from build123d import *

# Parameters (mm, degrees)
F1_DEPTH = 289.46
F2_W     = 128
F2_H     = 8.4
F3_DEPTH = 7
F5_DEPTH = 289.46


with BuildPart() as f1:
    # F0 (on Front) → F1 (new body)
    with BuildSketch(Plane.XZ):
        Polygon((-47.436745, 38.990075), (-57.436745, 38.990075), (-57.436745, 36.490075), (-54.436745, 36.490075), (-54.436745, 33.090075), (-56.436745, 33.090075), (-56.436745, 30.590075), (-47.436745, 30.590075), align=None)
    extrude(amount=F1_DEPTH)

    # F2 (on Front) → F3 (join)
    with BuildSketch(Plane.XZ):
        with Locations((-111.436745, 34.790075)):
            Rectangle(F2_W, F2_H)
    extrude(amount=-F3_DEPTH)

    # F4 (on Front) → F5 (join)
    with BuildSketch(Plane.XZ):
        Polygon((-165.436745, 36.57085), (-165.436745, 39.07085), (-175.436745, 39.07085), (-175.436745, 30.67085), (-166.436745, 30.67085), (-166.436745, 33.17085), (-168.436745, 33.17085), (-168.436745, 36.57085), align=None)
    extrude(amount=F5_DEPTH)


solid = f1.part
CAD build for the part. Positions are in the model's coordinates, mm. Round coordinates to 2 decimals unless told otherwise and drop trailing zeros. Write each loop counter-clockwise with the first axis right and the second up, starting at its lowest first coordinate (ties: lowest second). Pieces come first, ordered by that corner, then holes. Notation, with made-up numbers: M 20,17 L 49,17 A10 cw 49,27 Z; hole C 79,28 d6. An arc over 180 degrees is marked long. Use a Markdown table: item, result. Add a question column.
1. Slice it at B-B on z = 35. Give the cut face in (x, y).
2. Slice it at A-A on y = -19. Give the cut face in (x, z), then the cut area to 3 significant figures.
3. Slice it at C-C on x = -127.5. Give the cut face in (y, z), then the cut area to 3 significant figures.
4. Flat gauge pins, fed straight in: P1, Ø2.5, axis at x = -109, z = 34, coming from the -Y side; P2, Ø0.9, axis at x = -167.5, y = -157.5, coming from the -Z side; P3, Ø1.6, axis at x = -55.5, y = -91.5, coming from the +Z side. Where does each tip first touch, or does it go through?
5. Drill centre lines: probe 1 along X at (y, z) = (-88.5, 32.5); probe 2 along X at (y, z) = (-136, 38); probe 3 along Y at (x, z) = (-120.5, 32.75). Where is each one in solid material? Low to high.
6. Pull direction X, two halves, no side cores. Call faces 1 (the face through (-171, -143, 30.671)), 2 (the face through (-47.437, -143, 35)), 3 (the face through (-102, 0, 35)): released by +X, released by -X, zero draft, split by the parting line, or undercut.
Reply:
| question | item | result |
|---|---|---|
| 1 | outline | M -175.44,-289.46 L -168.44,-289.46 L -168.44,0 L -54.44,0 L -54.44,-289.46 L -47.44,-289.46 L -47.44,7 L -175.44,7 Z |
| 2 | outline | M -175.44,30.67 L -166.44,30.67 L -166.44,33.17 L -168.44,33.17 L -168.44,36.57 L -165.44,36.57 L -165.44,39.07 L -175.44,39.07 Z; M -57.44,36.49 L -54.44,36.49 L -54.44,33.09 L -56.44,33.09 L -56.44,30.59 L -47.44,30.59 L -47.44,38.99 L -57.44,38.99 Z |
| 2 | area | 143 mm^2 |
| 3 | outline | M 0,30.59 L 7,30.59 L 7,38.99 L 0,38.99 Z |
| 3 | area | 58.8 mm^2 |
| 4 | P1 | stops at y = 0 |
| 4 | P2 | stops at z = 30.67 |
| 4 | P3 | stops at z = 38.99 |
| 5 | probe 1 | x = -175.44 to -166.44, -56.44 to -47.44 |
| 5 | probe 2 | x = -175.44 to -165.44, -57.44 to -47.44 |
| 5 | probe 3 | y = 0 to 7 |
| 6 | face 1 | zero draft |
| 6 | face 2 | released by +X |
| 6 | face 3 | undercut |
